Source: CAD feature listing. Evaluate the final solid. Frame: model axes, mm. Face numbers are marked on the shaded views. Give positions to 0.01 mm unless a question says otherwise; leave off trailing zeros. Loops run counter-clockwise (first coordinate to the right, second up) from the corner with the lowest first, then second, coordinate; pieces in that order, holes last. Notation, with made-up numbers: M -4.5,9.5 L 48.5,9.5 A16 ccw 48.5,25.5 Z; hole C 85.5,43 d7. An arc over 180 degrees is marked long. Put each result on its own line as item: value.
from build123d import *

# Parameters (mm, degrees)
F2_DEPTH = 6
F0_R     = 16
F3_DEPTH = 415.3325557709
F0_R_2   = 8.745861022
F4_DEPTH = 8
F5_DEPTH = 13


with BuildPart() as f2:
    # F1 (on Top) → F2 (new body)
    with BuildSketch(Plane.XY):
        with BuildLine():
            Line((-12.8886751705, -28.5254933068), (0, -28.5254933068))
            Line((0, -28.5254933068), (12.8886751705, -28.5254933068))
            ThreePointArc((12.8886751705, -28.5254933068), (16.1500065629, -27.3154428512), (17.8327877404, -24.2709803264))
            Line((17.8327877404, -24.2709803264), (32.4659266708, 72.7768343533))
            ThreePointArc((32.4659266708, 72.7768343533), (29.0034375943, 84.7972895893), (17.6335889612, 90.0132954121))
            Line((17.6335889612, 90.0132954121), (0, 90.0132954121))
            Line((0, 90.0132954121), (-17.6335889612, 90.0132954121))
            ThreePointArc((-17.6335889612, 90.0132954121), (-29.0034375943, 84.7972895893), (-32.4659266708, 72.7768343533))
            Line((-32.4659266708, 72.7768343533), (-17.8327877404, -24.2709803264))
            ThreePointArc((-17.8327877404, -24.2709803264), (-16.1500065629, -27.3154428512), (-12.8886751705, -28.5254933068))
        make_face()
    extrude(amount=F2_DEPTH)

    # F0 (on Top) → F3 (join)
    with BuildSketch(Plane.XY):
        Circle(F0_R)
    extrude(amount=F3_DEPTH)

    # F0 (on Top) → F4 (join, symmetric)
    with BuildSketch(Plane.XY):
        with Locations((17.5, 75)):
            Circle(F0_R_2)
        with Locations((-17.5, 75)):
            Circle(F0_R_2)
    extrude(amount=F4_DEPTH, both=True)

    # F0 (on Top) → F5 (join)
    with BuildSketch(Plane.XY):
        Circle(F0_R)
    extrude(amount=-F5_DEPTH)


solid = f2.part
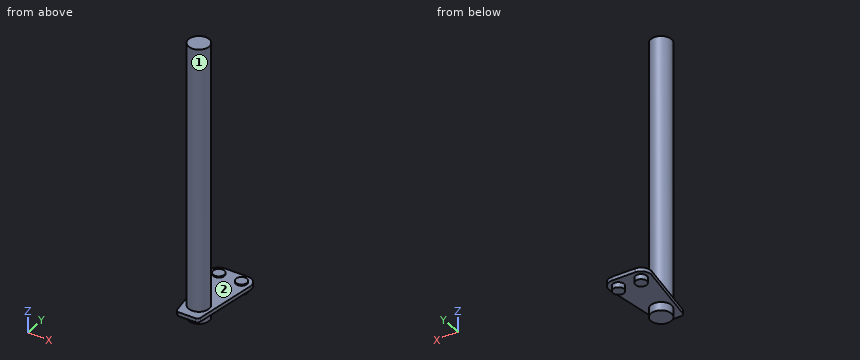
1. Section query C-C (z = 89.5). Output: boundary loops of the cut face in (x, y), plus the area to 3 significant figures.
Found:
outline: C 0,0 d32
area: 804 mm^2
2. Section query B-B (y = -10). Output: boundary loops of the cut face in (x, z), plus the area to 3 significant figures.
Found:
outline: M -19.98,0 L -12.49,0 L -12.49,-13 L 12.49,-13 L 12.49,0 L 19.98,0 L 19.98,6 L 12.49,6 L 12.49,415.33 L -12.49,415.33 L -12.49,6 L -19.98,6 Z
area: 10,800 mm^2
3. Section query A-A (x = 0). Output: boundary loops of the cut face in (y, z).
Found:
outline: M -28.53,0 L -16,0 L -16,-13 L 16,-13 L 16,0 L 90.01,0 L 90.01,6 L 16,6 L 16,415.33 L -16,415.33 L -16,6 L -28.53,6 Z
4. Contact query for flat-ended pins moving along their axis: P1, Ø14, axis at x = -18, y = 74, coming from the -Z side; P2, Ø12, axis at x = -2.5, z = 30.5, coming from the -Y side; P3, Ø10, axis at x = -14.5, z = 349, coming from the -Y side; P4, Ø19.5, axis at x = -12.5, y = 11, coming from the +Z side. Output: stop coordinate, or through.
Found:
P1: z = -8
P2: y = -16
P3: y = -12.87
P4: z = 415.33
5. Material intervals for line 1 (Z direction, x = 18, y = 37.5); line 2 (Z direction, x = -14, y = 78.5); line 3 (X direction, y = 1.5, z = 65.5), sorted ascending. Write a range as from..to.
Found:
line 1: 0..6
line 2: -8..8
line 3: -15.93..15.93
6. Draft query along Y for the marked faces 1 and 2. Return one class per face: pulls with the +Y half, pulls with the -Y half, needs draft (parallel to the pull), parting line crosses it, or undercut.
Found:
face 1: parting line crosses it
face 2: undercut
